Build history of the part. All positions in model axes, mm. Face numbers are marked on the shaded views. A direction names the side the tool comes from. Give positions to 0.01 mm unless a question says otherwise; leave off trailing zeros. Write each loop counter-clockwise with the first axis right and the second up, starting at its lowest first coordinate (ties: lowest second). Pieces come first, ordered by that corner, then holes.
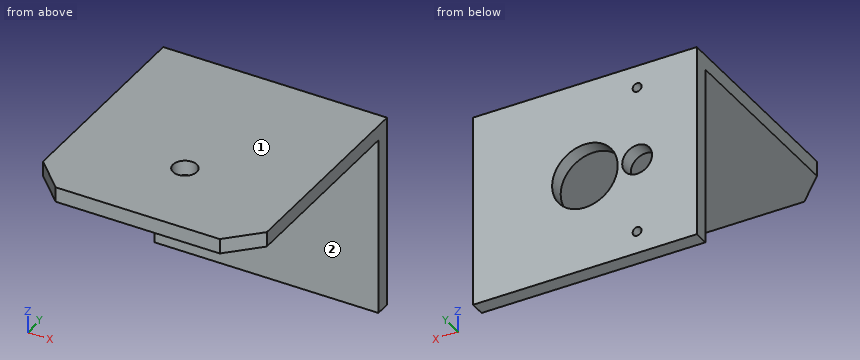
from build123d import *

# Parameters (mm, degrees)
SKETCH1_W           = 75
SKETCH1_H           = 65
SKETCH1_R           = 5
SKETCH1_R_2         = 11
SKETCH1_R_3         = 1.5
BOSS_EXTRUDE1_DEPTH = 5
SKETCH2_W           = 75
SKETCH2_H           = 5
BOSS_EXTRUDE2_DEPTH = 75
CUT_EXTRUDE1_REACH  = 67
CUT_EXTRUDE2_REACH  = 7
CUT_EXTRUDE3_REACH  = 67
SKETCH5_R           = 4
CUT_EXTRUDE4_REACH  = 67
SKETCH6_R           = 2.5
CUT_EXTRUDE5_REACH  = 7


with BuildPart() as part:
    # Sketch1 → Boss-Extrude1 (new body)
    with BuildSketch(Plane(origin=(0, 0, 0), x_dir=(1, 0, 0), z_dir=(0, 1, 0))):
        Rectangle(SKETCH1_W, SKETCH1_H)
        with Locations((-17.5, 0)):
            Circle(SKETCH1_R, mode=Mode.SUBTRACT)
        Circle(SKETCH1_R_2, mode=Mode.SUBTRACT)
        with Locations((-17.5, -25)):
            Circle(SKETCH1_R_3, mode=Mode.SUBTRACT)
        with Locations((-17.5, 25)):
            Circle(SKETCH1_R_3, mode=Mode.SUBTRACT)
    extrude(amount=BOSS_EXTRUDE1_DEPTH)

    # Sketch2 → Boss-Extrude2 (add)
    with BuildSketch(Plane.XZ):
        with Locations((0, 30)):
            Rectangle(SKETCH2_W, SKETCH2_H)
        with Locations((0, -30)):
            Rectangle(SKETCH2_W, SKETCH2_H)
    extrude(amount=BOSS_EXTRUDE2_DEPTH)

    # Sketch3 → Cut-Extrude1 (cut, up to next)
    with BuildSketch(Plane.XY.offset(32.5), mode=Mode.PRIVATE) as cut_extrude1_sk1:
        Polygon((-37.5, -75), (-27.5, -75), (-37.5, -65), align=None)
    cut_extrude1_tool1 = extrude(cut_extrude1_sk1.sketch, amount=-CUT_EXTRUDE1_REACH, mode=Mode.PRIVATE) & part.part
    add(cut_extrude1_tool1.solids().sort_by_distance((-34.166667, -71.666667, 32.5))[0], mode=Mode.SUBTRACT)
    # Sketch3 → Cut-Extrude1 (cut, up to next)
    with BuildSketch(Plane.XY.offset(32.5), mode=Mode.PRIVATE) as cut_extrude1_sk2:
        Polygon((37.5, -75), (37.5, -65), (27.5, -75), align=None)
    cut_extrude1_tool2 = extrude(cut_extrude1_sk2.sketch, amount=-CUT_EXTRUDE1_REACH, mode=Mode.PRIVATE) & part.part
    add(cut_extrude1_tool2.solids().sort_by_distance((34.166667, -71.666667, 32.5))[0], mode=Mode.SUBTRACT)

    # Sketch4 → Cut-Extrude2 (cut, up to next)
    with BuildSketch(Plane.XY.offset(-27.5), mode=Mode.PRIVATE) as cut_extrude2_sk1:
        Polygon((-37.5, -65), (-37.5, -75), (-27.5, -75), align=None)
    cut_extrude2_tool1 = extrude(cut_extrude2_sk1.sketch, amount=-CUT_EXTRUDE2_REACH, mode=Mode.PRIVATE) & part.part
    add(cut_extrude2_tool1.solids().sort_by_distance((-34.166667, -71.666667, -27.5))[0], mode=Mode.SUBTRACT)
    # Sketch4 → Cut-Extrude2 (cut, up to next)
    with BuildSketch(Plane.XY.offset(-27.5), mode=Mode.PRIVATE) as cut_extrude2_sk2:
        Polygon((37.5, -65), (27.5, -75), (37.5, -75), align=None)
    cut_extrude2_tool2 = extrude(cut_extrude2_sk2.sketch, amount=-CUT_EXTRUDE2_REACH, mode=Mode.PRIVATE) & part.part
    add(cut_extrude2_tool2.solids().sort_by_distance((34.166667, -71.666667, -27.5))[0], mode=Mode.SUBTRACT)

    # Sketch5 → Cut-Extrude3 (cut, up to next)
    with BuildSketch(Plane.XY.offset(32.5), mode=Mode.PRIVATE) as cut_extrude3_sk1:
        with Locations((0, -47.5)):
            Circle(SKETCH5_R)
    cut_extrude3_tool1 = extrude(cut_extrude3_sk1.sketch, amount=-CUT_EXTRUDE3_REACH, mode=Mode.PRIVATE) & part.part
    add(cut_extrude3_tool1.solids().sort_by_distance((0, -47.5, 32.5))[0], mode=Mode.SUBTRACT)

    # Sketch6 → Cut-Extrude4 (cut, up to next)
    with BuildSketch(Plane(origin=(0, 0, -32.5), x_dir=(-1, 0, 0), z_dir=(0, 0, -1)), mode=Mode.PRIVATE) as cut_extrude4_sk1:
        with Locations((0, -47.5)):
            Circle(SKETCH6_R)
    cut_extrude4_tool1 = extrude(cut_extrude4_sk1.sketch, amount=-CUT_EXTRUDE4_REACH, mode=Mode.PRIVATE) & part.part
    add(cut_extrude4_tool1.solids().sort_by_distance((0, -47.5, -32.5))[0], mode=Mode.SUBTRACT)

    # Sketch7 → Cut-Extrude5 (cut, up to next)
    with BuildSketch(Plane.XY.offset(-27.5), mode=Mode.PRIVATE) as cut_extrude5_sk1:
        Polygon((-37.5, 0), (37.5, 0), (37.5, -65), (27.5, -75), (-27.5, -75), (-37.5, -65), align=None)
    cut_extrude5_tool1 = extrude(cut_extrude5_sk1.sketch, amount=-CUT_EXTRUDE5_REACH, mode=Mode.PRIVATE) & part.part
    add(cut_extrude5_tool1.solids().sort_by_distance((0, -36.881599, -27.5))[0], mode=Mode.SUBTRACT)


solid = part.part
1. Saw through at A-A on z = 25. Give the cut face in (x, y), plus the area to 3 significant figures.
2. Drill centre lines: line 1 along Z through (x, y) = (-17.5, 2.45); line 2 along X through (y, z) = (2, 0); line 3 along Y through (x, z) = (0, 28). Where is each one in solid material? Low to high.
3. Saw through at C-C on y = -47.5. Give the cut face in (x, z), plus the area to 3 significant figures.
4. 3-axis set-ups, long thin cutter, end or side, ignore diameter. For the marked faces 1 and 2: which of +Z, -Z, +X, -X, +Y, -Y reach the whole face in a straight line?
5. Saw through at D-D on z = 0. Give the cut face in (x, y).
6. Saw through at B-B on x = 0. Give the cut face in (y, z).
7. Drop flat-ended pins along their axis: pin 1 (10 mm diameter, centred on x = -22.5, y = -32, fed in from -Z); pin 2 (1 mm diameter, centred on x = -3.5, z = -16, fed in from -Y). Give the stop position or say it passes through.
Outcome:
1. outline: (-37.5, 0) - (-19, 0) - (-19, 5) - (-37.5, 5) - close; (-16, 0) - (37.5, 0) - (37.5, 5) - (-16, 5) - close
1. area: 360 mm2
2. line 1: z = -32.5 to -26.5, -23.5 to -5, 5 to 23.5, 26.5 to 32.5
2. line 2: x = -37.5 to -22.5, -12.5 to -11, 11 to 37.5
2. line 3: y = -75 to -51.5, -43.5 to 5
3. outline: (-37.5, 27.5) - (-4, 27.5) - (-4, 32.5) - (-37.5, 32.5) - close; (4, 27.5) - (37.5, 27.5) - (37.5, 32.5) - (4, 32.5) - close
3. area: 335 mm2
4. face 1: +Z, +X, -X, +Y, -Y
4. face 2: -Z, +X, -X, -Y
5. outline: (-37.5, 0) - (-22.5, 0) - (-22.5, 5) - (-37.5, 5) - close; (-12.5, 0) - (-11, 0) - (-11, 5) - (-12.5, 5) - close; (11, 0) - (37.5, 0) - (37.5, 5) - (11, 5) - close
6. outline: (-75, 27.5) - (-51.5, 27.5) - (-51.5, 32.5) - (-75, 32.5) - close; (-43.5, 27.5) - (0, 27.5) - (0, 11) - (5, 11) - (5, 32.5) - (-43.5, 32.5) - close; (0, -32.5) - (5, -32.5) - (5, -11) - (0, -11) - close
7. pin 1: stops at z = 27.5
7. pin 2: stops at y = 0
